from build123d import *

# Parameters (mm, degrees)
F0_R     = 12.7
F1_DEPTH = 10.16
F2_W     = 3.175
F2_H     = 3.175
F3_DEPTH = 7.62
F4_R     = 2.7305
F5_DEPTH = 12.7


with BuildPart() as f1:
    # F0 (on Top) → F1 (new body, symmetric)
    with BuildSketch(Plane.XY):
        Circle(F0_R)
    extrude(amount=F1_DEPTH, both=True)

    # F2 (on face) → F3 (cut, symmetric)
    with BuildSketch(Plane.XY.offset(10.16)):
        with Locations((-1.5875, 1.5875)):
            Rectangle(F2_W, F2_H)
        with Locations((1.5875, 1.5875)):
            Rectangle(F2_W, F2_H)
        with Locations((-1.5875, -1.5875)):
            Rectangle(F2_W, F2_H)
        with Locations((1.5875, -1.5875)):
            Rectangle(F2_W, F2_H)
    extrude(amount=F3_DEPTH, both=True, mode=Mode.SUBTRACT)

    # F4 (on face) → F5 (cut, symmetric)
    with BuildSketch(Plane(origin=(0, 0, -10.16), x_dir=(1, 0, 0), z_dir=(0, 0, -1))):
        Circle(F4_R)
    extrude(amount=F5_DEPTH, both=True, mode=Mode.SUBTRACT)


solid = f1.part
Here's how the part is built. I have some questions about the finished solid (model axes, mm). A direction names the side the tool comes from. Round coordinates to 2 decimals unless told otherwise and drop trailing zeros. Loops run counter-clockwise (first coordinate to the right, second up) from the corner with the lowest first, then second, coordinate; pieces in that order, holes last.
1. If we section it at A-A on y = 0: Write out the boundary of the cut face in (x, z) (1 decimal).
Answer list:
outline: (-12.7, -10.2) - (-2.7, -10.2) - (-2.7, 2.5) - (-3.2, 2.5) - (-3.2, 10.2) - (-12.7, 10.2) - close; (2.7, -10.2) - (12.7, -10.2) - (12.7, 10.2) - (3.2, 10.2) - (3.2, 2.5) - (2.7, 2.5) - close
2. If we section it at D-D on z = -0.5: Write out the boundary of the cut face in (x, y), plus the area to 3 significant figures.
Answer list:
outline: circle Ø25.4 at (0, 0); hole circle Ø5.46 at (0, 0)
area: 483 mm2
3. If we section it at B-B on z = 4.75: Write out the boundary of the cut face in (x, y) (3 decimals).
Answer list:
outline: circle Ø25.4 at (0, 0); hole (-3.175, -3.175) - (3.175, -3.175) - (3.175, 3.175) - (-3.175, 3.175) - close
4. If I drill on line 1 along Y through (x, z) = (0, -5.5); line 2 along X through (y, z) = (-2.5, -2); line 3 along Y through (x, z) = (1.75, 8) (3 decimals), over which ranges is the centre line in solid material (lowest first)?
Answer list:
line 1: y = -12.7 to -2.73, 2.73 to 12.7
line 2: x = -12.45 to -1.1, 1.1 to 12.45
line 3: y = -12.579 to -3.175, 3.175 to 12.579
5. Which directions (+Z, -Z, +X, -X, +Y, -Y) give clear straight access to the entire face, cutting with the end or side of a thin tool? Please do faces 1 (the face through (3, 0, 2.54)), 2 (the face through (0, 3, -10.16)).
Answer list:
face 1: +Z
face 2: -Z, +X, -X, +Y, -Y
6. For P1, Ø2, axis at x = 2.5, z = -5, coming from the +Y side; P2, Ø1, axis at x = 4.5, z = 5, coming from the -Y side; P3, Ø5, axis at y = 7, z = -1.5, coming from the +X side, each with a flat end and sliding along its axis, tell me the tip position at first contact or that it passes through.
Answer list:
P1: stops at y = 12.61
P2: stops at y = -12.05
P3: stops at x = 11.88
7. We'd pull the mould along X, two halves only. Please class faces 3 (the face through (-2.75, -12.4, 0.14)), 4 (the face through (5, 0, 10.16)), 5 (the face through (2.604, -0.82, -3.899)): +X half, -X half, draft (parallel to the pull), parting line (faces both ways), or undercut.
Answer list:
face 3: parting line
face 4: draft
face 5: undercut
